Here's the drawing with two shaded views (mm, measured from the low corner). I have some questions. Round coordinates to 2 decimals unless told otherwise and drop trailing zeros. Order: outer loops, then holes, each group sorted by start corner. A loop starts at its lowest first (then second) coordinate and runs counter-clockwise, first axis right, second up. Notation, with made-up numbers: (8, 52.5) - (60, 52.5) arc R18 cw to (60, 83.5) - close; hole circle Ø2 at (26.5, -37.75). An arc over 180 degrees is marked (long way). One line per item, written item: value.
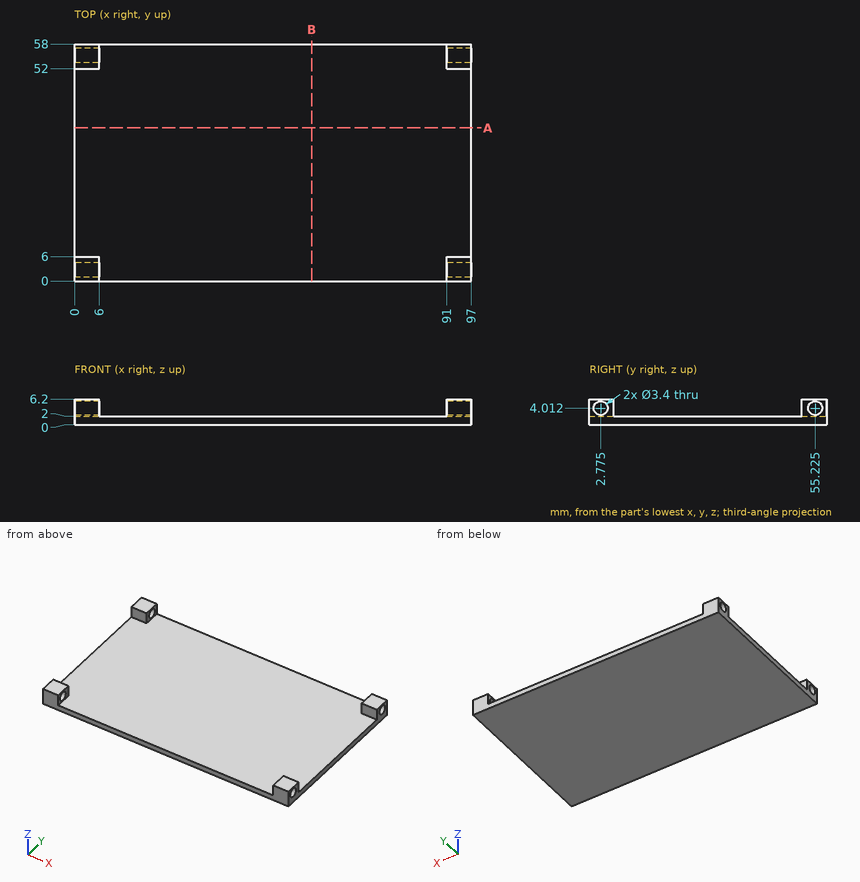
Q1. If we section it at A-A, the plane y = 37.5: Please give me the cut outline in (x, z).
Results list:
outline: (0, 0) - (97, 0) - (97, 2) - (0, 2) - close
Q2. If we section it at B-B, the plane x = 58: Please give me the cut outline in (y, z).
Results list:
outline: (0, 0) - (58, 0) - (58, 2) - (0, 2) - close
Q3. If I drill on line 1 along Y through (x, z) = (91.5, 5.25); line 2 along X through (y, z) = (3.5, 6); line 3 along Z through (x, y) = (63, 13.5), over which ranges is the centre line in solid material (lowest first)?
Results list:
line 1: 0 to 1.61, 3.94 to 6, 52 to 54.06, 56.39 to 58
line 2: 0 to 6, 91 to 97
line 3: 0 to 2
